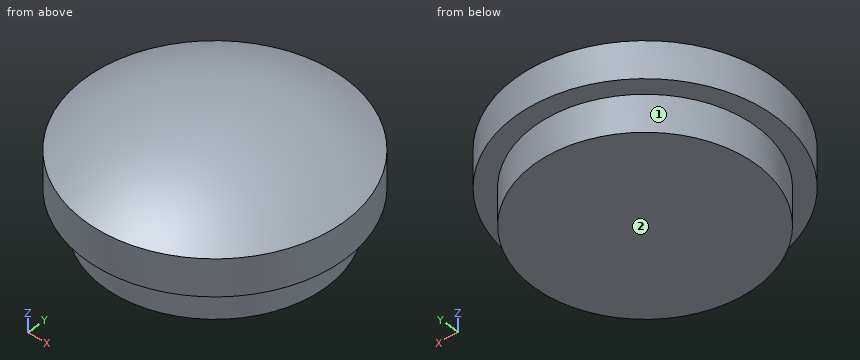
from build123d import *

# Parameters (mm, degrees)
SKETCH1_R         = 7.62
EXTRUDE1_DEPTH    = 2.54
SKETCH2_R         = 8.89
EXTRUDE2_DEPTH    = 2.54
DOME1_FACE_RADIUS = 8.89
DOME1_HEIGHT      = 2.54


with BuildPart() as part:
    # Sketch1 → Extrude1 (new body)
    with BuildSketch(Plane.XY):
        Circle(SKETCH1_R)
    extrude(amount=EXTRUDE1_DEPTH)

    # Sketch2 → Extrude2 (add)
    with BuildSketch(Plane.XY.offset(2.54)):
        Circle(SKETCH2_R)
    extrude(amount=EXTRUDE2_DEPTH)

    # Dome1: a dome of height H over a round flat face of radius A is a cap of a sphere of radius (A * A + H * H) / (2 * H)
    dome1_r = (DOME1_FACE_RADIUS * DOME1_FACE_RADIUS + DOME1_HEIGHT * DOME1_HEIGHT) / (2 * DOME1_HEIGHT)
    dome1_base = Plane((0, 0, 5.08), z_dir=(0, 0, 1))
    with Locations(dome1_base.offset(DOME1_HEIGHT - dome1_r)):
        dome1_ball = Sphere(dome1_r, mode=Mode.PRIVATE)
    add(split(dome1_ball, bisect_by=dome1_base, keep=Keep.TOP, mode=Mode.PRIVATE))


solid = part.part
Source: CAD feature listing. Evaluate the final solid. Frame: model axes, mm. Face numbers are marked on the shaded views. A direction names the side the tool comes from. Give positions to 0.01 mm unless a question says otherwise; leave off trailing zeros. Write each loop counter-clockwise with the first axis right and the second up, starting at its lowest first coordinate (ties: lowest second). Pieces come first, ordered by that corner, then holes. Notation, with made-up numbers: (27.25, 0) - (37.25, 0) arc R11 ccw to (37.25, 19) - close; hole circle Ø3 at (36.25, 66.5). An arc over 180 degrees is marked (long way). Write item = value, one per line. Start each with the question number.
Q1. Cut plane A-A, the plane x = 0. Return loops of the section in (y, z) (1 decimal), then the cut area to 3 significant figures.
Q2. Pin query (flat end, axial travel): pin 1 Ø1.5 at (x, z) = (-2.5, 5) entering from +Y; pin 2 Ø2 at (x, y) = (-5, 2.5) entering from +Z; pin 3 Ø2 at (x, y) = (5, 7) entering from +Z. Return the tip coordinate at first contact, or that it passes through.
Q3. Material intervals for probe 1 along X at (y, z) = (-3, 4.5); probe 2 along Y at (x, z) = (-7, 4.5); probe 3 along Y at (x, z) = (0, 5.5), sorted ascending.
Q4. Cut plane D-D, the plane z = 5.5. Return loops of the section in (x, y).
Q5. Reachability of the marked faces 1 and 2 from +Z, -Z, +X, -X, +Y, -Y: full face, straight path, thin tool, end or side. Return the list, or none.
Q6. Cut plane C-C, the plane z = 1.25. Return loops of the section in (x, y).
Computed values:
q1.outline = (-8.9, 2.5) - (-7.6, 2.5) - (-7.6, 0) - (7.6, 0) - (7.6, 2.5) - (8.9, 2.5) - (8.9, 5.1) arc R16.8 ccw to (-8.9, 5.1) - close
q1.area = 114 mm²
q2.pin_1 = 8.72
q2.pin_2 = 6.98
q2.pin_3 = 5.8
q3.probe_1 = -8.37 to 8.37
q3.probe_2 = -5.48 to 5.48
q3.probe_3 = -8.18 to 8.18
q4.outline = circle Ø16.35 at (0, 0)
q5.face_1 = -Z
q5.face_2 = -Z, +X, -X, +Y, -Y
q6.outline = circle Ø15.24 at (0, 0)
